Read the model definition and answer for the solid it produces. Units are mm, in the model's axes. Round coordinates to 2 decimals unless told otherwise and drop trailing zeros. Order: outer loops, then holes, each group sorted by start corner. A loop starts at its lowest first (then second) coordinate and runs counter-clockwise, first axis right, second up. Notation, with made-up numbers: (-24, 16.5) -> (-2, 16.5) arc R21 ccw to (-2, 23.5) -> close; hole circle Ø9 at (30, 87). An arc over 180 degrees is marked (long way). One line per item, written item: value. Start each with the question number.
1. Section B-B (x = 72.55) is taken. Give the vertices of the cut face in (y, z) (3 decimals).
2. The mould has two halves that part along X. Classify faces 1 (the face through (-1, 0, -2)), 2 (the face through (69.95, 3.22, -98.53)), 3 (the face through (82.55, 3, 1)): released by +X, released by -X, zero draft, split by the parting line, or undercut.
3. A flat-ended cylindrical pin translates along its axis: pin 1 Ø3 at (x, z) = (72.55, 97.95) entering from +Y. Find the tip coordinate at first contact, or state that the pin passes through.
4. Section A-A (z = 97.95) is taken. Give the vertices of the cut face in (x, y) (3 decimals), then the cut area to 3 significant figures.
5. Consider line 1 (Z direction, x = -43.5, y = 1); line 2 (X direction, y = 5, z = -97.95) (3 decimals); line 3 (Z direction, x = -73.5, y = 2). Determine where each line is inside the solid, lowest interval first.
from build123d import *

# Parameters (mm, degrees)
SKETCH1_W           = 165.1
SKETCH1_H           = 215.9
BOSS_EXTRUDE1_DEPTH = 6.35
CUT_EXTRUDE2_REACH  = 138.044
SKETCH3_R           = 2.665
FILLET1_R           = 2.54
CUT_EXTRUDE3_REACH  = 138.044
SKETCH2_R           = 4.7625
SKETCH2_R_2         = 4.5


with BuildPart() as part:
    # Sketch1 → Boss-Extrude1 (new body)
    with BuildSketch(Plane(origin=(0, 0, 0), x_dir=(1, 0, 0), z_dir=(0, 1, 0))):
        Rectangle(SKETCH1_W, SKETCH1_H)
    extrude(amount=BOSS_EXTRUDE1_DEPTH)

    # Sketch3 → Cut-Extrude2 (cut, up to next)
    with BuildSketch(Plane(origin=(0, 6.35, 0), x_dir=(-1, 0, 0), z_dir=(0, 1, 0)), mode=Mode.PRIVATE) as cut_extrude2_sk1:
        with Locations(Location((72.55, 97.95, 0), (0, 0, 90))):
            Circle(SKETCH3_R)
    cut_extrude2_tool1 = extrude(cut_extrude2_sk1.sketch, amount=-CUT_EXTRUDE2_REACH, mode=Mode.PRIVATE) & part.part
    # Sketch3 → Cut-Extrude2 (cut, up to next)
    with BuildSketch(Plane(origin=(0, 6.35, 0), x_dir=(-1, 0, 0), z_dir=(0, 1, 0)), mode=Mode.PRIVATE) as cut_extrude2_sk2:
        with Locations(Location((-72.55, 97.95, 0), (0, 0, 90))):
            Circle(SKETCH3_R)
    cut_extrude2_tool2 = extrude(cut_extrude2_sk2.sketch, amount=-CUT_EXTRUDE2_REACH, mode=Mode.PRIVATE) & part.part
    # Sketch3 → Cut-Extrude2 (cut, up to next)
    with BuildSketch(Plane(origin=(0, 6.35, 0), x_dir=(-1, 0, 0), z_dir=(0, 1, 0)), mode=Mode.PRIVATE) as cut_extrude2_sk3:
        with Locations(Location((-72.55, -97.95, 0), (0, 0, 90))):
            Circle(SKETCH3_R)
    cut_extrude2_tool3 = extrude(cut_extrude2_sk3.sketch, amount=-CUT_EXTRUDE2_REACH, mode=Mode.PRIVATE) & part.part
    # Sketch3 → Cut-Extrude2 (cut, up to next)
    with BuildSketch(Plane(origin=(0, 6.35, 0), x_dir=(-1, 0, 0), z_dir=(0, 1, 0)), mode=Mode.PRIVATE) as cut_extrude2_sk4:
        with Locations(Location((72.55, -97.95, 0), (0, 0, 90))):
            Circle(SKETCH3_R)
    cut_extrude2_tool4 = extrude(cut_extrude2_sk4.sketch, amount=-CUT_EXTRUDE2_REACH, mode=Mode.PRIVATE) & part.part
    add(cut_extrude2_tool1.solids().sort_by_distance((-72.55, 6.35, 97.95))[0], mode=Mode.SUBTRACT)
    add(cut_extrude2_tool2.solids().sort_by_distance((72.55, 6.35, 97.95))[0], mode=Mode.SUBTRACT)
    add(cut_extrude2_tool3.solids().sort_by_distance((72.55, 6.35, -97.95))[0], mode=Mode.SUBTRACT)
    add(cut_extrude2_tool4.solids().sort_by_distance((-72.55, 6.35, -97.95))[0], mode=Mode.SUBTRACT)

    # Fillet1
    fillet1_edges = [part.edges().sort_by_distance(p)[0] for p in [
        (-82.55, 3.175, -107.95),
        (82.55, 3.175, -107.95),
        (82.55, 3.175, 107.95),
        (-82.55, 3.175, 107.95),
    ]]
    fillet(fillet1_edges, radius=FILLET1_R)

    # Sketch2 → Cut-Extrude3 (cut, up to next)
    with BuildSketch(Plane(origin=(0, 6.35, 0), x_dir=(1, 0, 0), z_dir=(0, 1, 0)), mode=Mode.PRIVATE) as cut_extrude3_sk1:
        with Locations(Location((-42.8625, 80.9625, 0), (0, 0, 270))):
            Circle(SKETCH2_R)
    cut_extrude3_tool1 = extrude(cut_extrude3_sk1.sketch, amount=-CUT_EXTRUDE3_REACH, mode=Mode.PRIVATE) & part.part
    # Sketch2 → Cut-Extrude3 (cut, up to next)
    with BuildSketch(Plane(origin=(0, 6.35, 0), x_dir=(1, 0, 0), z_dir=(0, 1, 0)), mode=Mode.PRIVATE) as cut_extrude3_sk2:
        with Locations(Location((-42.8625, -80.9625, 0), (0, 0, 270))):
            Circle(SKETCH2_R_2)
    cut_extrude3_tool2 = extrude(cut_extrude3_sk2.sketch, amount=-CUT_EXTRUDE3_REACH, mode=Mode.PRIVATE) & part.part
    # Sketch2 → Cut-Extrude3 (cut, up to next)
    with BuildSketch(Plane(origin=(0, 6.35, 0), x_dir=(1, 0, 0), z_dir=(0, 1, 0)), mode=Mode.PRIVATE) as cut_extrude3_sk3:
        with Locations(Location((42.8625, -80.9625, 0), (0, 0, 270))):
            Circle(SKETCH2_R_2)
    cut_extrude3_tool3 = extrude(cut_extrude3_sk3.sketch, amount=-CUT_EXTRUDE3_REACH, mode=Mode.PRIVATE) & part.part
    # Sketch2 → Cut-Extrude3 (cut, up to next)
    with BuildSketch(Plane(origin=(0, 6.35, 0), x_dir=(1, 0, 0), z_dir=(0, 1, 0)), mode=Mode.PRIVATE) as cut_extrude3_sk4:
        with Locations(Location((42.8625, 80.9625, 0), (0, 0, 270))):
            Circle(SKETCH2_R_2)
    cut_extrude3_tool4 = extrude(cut_extrude3_sk4.sketch, amount=-CUT_EXTRUDE3_REACH, mode=Mode.PRIVATE) & part.part
    add(cut_extrude3_tool1.solids().sort_by_distance((-42.8625, 6.35, -80.9625))[0], mode=Mode.SUBTRACT)
    add(cut_extrude3_tool2.solids().sort_by_distance((-42.8625, 6.35, 80.9625))[0], mode=Mode.SUBTRACT)
    add(cut_extrude3_tool3.solids().sort_by_distance((42.8625, 6.35, 80.9625))[0], mode=Mode.SUBTRACT)
    add(cut_extrude3_tool4.solids().sort_by_distance((42.8625, 6.35, -80.9625))[0], mode=Mode.SUBTRACT)


solid = part.part
Answer:
1. outline: (0, -107.95) -> (6.35, -107.95) -> (6.35, -100.615) -> (0, -100.615) -> close; (0, -95.285) -> (6.35, -95.285) -> (6.35, 95.285) -> (0, 95.285) -> close; (0, 100.615) -> (6.35, 100.615) -> (6.35, 107.95) -> (0, 107.95) -> close
2. face 1: zero draft
2. face 2: undercut
2. face 3: released by +X
3. pin 1: through
4. outline: (-82.55, 0) -> (-75.215, 0) -> (-75.215, 6.35) -> (-82.55, 6.35) -> close; (-69.885, 0) -> (69.885, 0) -> (69.885, 6.35) -> (-69.885, 6.35) -> close; (75.215, 0) -> (82.55, 0) -> (82.55, 6.35) -> (75.215, 6.35) -> close
4. area: 981 mm^2
5. line 1: -107.95 to -85.68, -76.24 to 76.51, 85.42 to 107.95
5. line 2: -82.55 to -75.215, -69.885 to 69.885, 75.215 to 82.55
5. line 3: -107.95 to -100.44, -95.46 to 95.46, 100.44 to 107.95
